Geometry check sheet. Reference: the model listing, model coordinates, mm. Face numbers are marked on the shaded views. Coordinates: 2 decimals unless noted, no trailing zeros. Loops run counter-clockwise (first coordinate to the right, second up) from the corner with the lowest first, then second, coordinate; pieces in that order, holes last. Notation, with made-up numbers: (73, -1.75) -> (84, -1.75) arc R36 cw to (84, 37.25) -> close; hole circle Ø10 at (21, -29). An arc over 180 degrees is marked (long way). Answer as a JSON object with one key per item and string values.
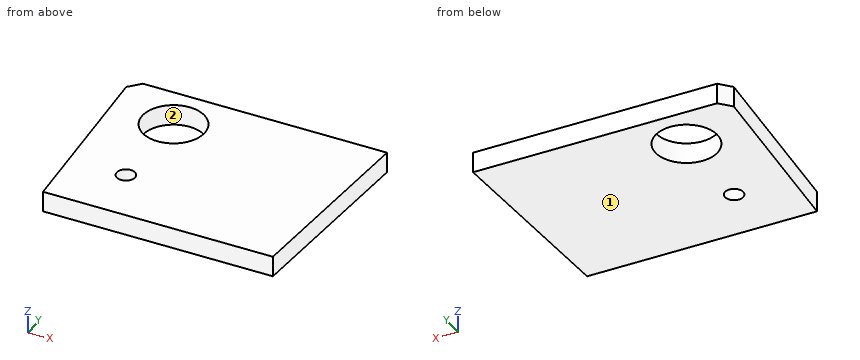
from build123d import *

# Parameters (mm, degrees)
SKETCH1_R             = 0.396875
SKETCH1_R_2           = 1.3462
EXTRUDE1_DEPTH        = 0.9
CHAMFER1_SIZE         = 1.3
CHAMFER1_SIZE2        = 1.136906158
CHAMFER1_EDGE_2_SIZE  = 1.3
CHAMFER1_EDGE_2_SIZE2 = 1.136906158
SKETCH2_R             = 0.396875
SKETCH2_R_2           = 1.3462
EXTRUDE2_DEPTH        = 0.9
CUT_EXTRUDE2_DEPTH    = 1.9
CHAMFER2_SIZE         = 0.5


with BuildPart() as part:
    # Sketch1 → Extrude1 (new body)
    with BuildSketch(Plane.XY):
        Polygon((-2.158886106, 43.490401799), (2.158886106, 43.490401799), (0.81962306, 34.990401799), (-0.81962306, 34.990401799), align=None)
        with Locations((0, 37.5)):
            Circle(SKETCH1_R, mode=Mode.SUBTRACT)
        with Locations((0, 41.5)):
            Circle(SKETCH1_R_2, mode=Mode.SUBTRACT)
    extrude(amount=EXTRUDE1_DEPTH)

    # Chamfer1
    chamfer1_edges = [part.edges().sort_by_distance(p)[0] for p in [
        (-2.158886106, 43.490401799, 0.45),
    ]]
    chamfer1_side = [part.faces().sort_by_distance(p)[0] for p in [
        (0, 43.490401799, 0.45),
    ]]
    chamfer(chamfer1_edges, length=CHAMFER1_SIZE, length2=CHAMFER1_SIZE2, reference=chamfer1_side[0])

    # Chamfer1 edge 2
    chamfer1_edge_2_edges = [part.edges().sort_by_distance(p)[0] for p in [
        (2.158886106, 43.490401799, 0.45),
    ]]
    chamfer1_edge_2_side = [part.faces().sort_by_distance(p)[0] for p in [
        (0, 43.490401799, 0.45),
    ]]
    chamfer(chamfer1_edge_2_edges, length=CHAMFER1_EDGE_2_SIZE, length2=CHAMFER1_EDGE_2_SIZE2, reference=chamfer1_edge_2_side[0])

    # Sketch2 → Extrude2 (add)
    with BuildSketch(Plane(origin=(0, 0, 0.9), x_dir=(-1, 0, 0), z_dir=(0, 0, -1))):
        Polygon((-8.212619969, 43.490401799), (8.212619969, 43.490401799), (7.655500535, 34.990401799), (-7.655500535, 34.990401799), align=None)
        with Locations(Location((0, 37.5, 0), (0, 0, 180))):  # turned: the seam where the file's is
            Circle(SKETCH2_R, mode=Mode.SUBTRACT)
        with Locations(Location((0, 41.5, 0), (0, 0, 180))):  # turned: the seam where the file's is
            Circle(SKETCH2_R_2, mode=Mode.SUBTRACT)
    extrude(amount=EXTRUDE2_DEPTH)

    # Sketch4 → Cut-Extrude2 (cut, through all)
    with BuildSketch(Plane(origin=(0, 0, 0), x_dir=(-1, 0, 0), z_dir=(0, 0, -1))):
        Polygon((2.293392099, 34.990401799), (2.850511533, 43.490401799), (8.212619969, 43.490401799), (7.655500535, 34.990401799), align=None)
    extrude(amount=-CUT_EXTRUDE2_DEPTH, mode=Mode.SUBTRACT)

    # Chamfer2
    chamfer2_edges = [part.edges().sort_by_distance(p)[0] for p in [
        (-2.850511533, 43.490401799, 0.45),
    ]]
    chamfer(chamfer2_edges, length=CHAMFER2_SIZE)


solid = part.part
1. Mould release check, pull along X, two halves, no side actions. Record for the marked faces 1 and 2: released by +X, released by -X, zero draft, split by the parting line, or undercut.
Evaluation:
{"face 1": "zero draft", "face 2": "undercut"}
2. Section check C-C, the plane y = 41.5. Record the boundary of the cut face in (x, z).
Evaluation:
{"outline": "(-2.72, 0) -> (-1.35, 0) -> (-1.35, 0.9) -> (-2.72, 0.9) -> close; (1.35, 0) -> (8.08, 0) -> (8.08, 0.9) -> (1.35, 0.9) -> close"}
3. Section check A-A, the plane x = 0. Record the boundary of the cut face in (y, z).
Evaluation:
{"outline": "(34.99, 0) -> (37.1, 0) -> (37.1, 0.9) -> (34.99, 0.9) -> close; (37.9, 0) -> (40.15, 0) -> (40.15, 0.9) -> (37.9, 0.9) -> close; (42.85, 0) -> (43.49, 0) -> (43.49, 0.9) -> (42.85, 0.9) -> close"}
4. Section check D-D, the plane y = 37.75. Record the boundary of the cut face in (x, z), then the cut area to 3 significant figures.
Evaluation:
{"outline": "(-2.47, 0) -> (-0.31, 0) -> (-0.31, 0.9) -> (-2.47, 0.9) -> close; (0.31, 0) -> (7.84, 0) -> (7.84, 0.9) -> (0.31, 0.9) -> close", "area": "8.72 mm^2"}
5. Thickness scan on probe 1 along Y at (x, z) = (0, 0.55); probe 2 along X at (y, z) = (37.5, 0.4); probe 3 along Y at (x, z) = (-0.75, 0.55). Record the ranges inside material, lowest first. Write a range as from..to.
Evaluation:
{"probe 1": "y = 34.99..37.1, 37.9..40.15, 42.85..43.49", "probe 2": "x = -2.46..-0.4, 0.4..7.82", "probe 3": "y = 34.99..40.38, 42.62..43.49"}
6. Section check B-B, the plane z = 0.6. Record the boundary of the cut face in (x, y), then the cut area to 3 significant figures.
Evaluation:
{"outline": "(-2.82, 42.99) -> (-2.29, 34.99) -> (7.66, 34.99) -> (8.21, 43.49) -> (-2.35, 43.49) -> close; hole circle Ø2.69 at (0, 41.5); hole circle Ø0.79 at (0, 37.5)", "area": "83.0 mm^2"}
